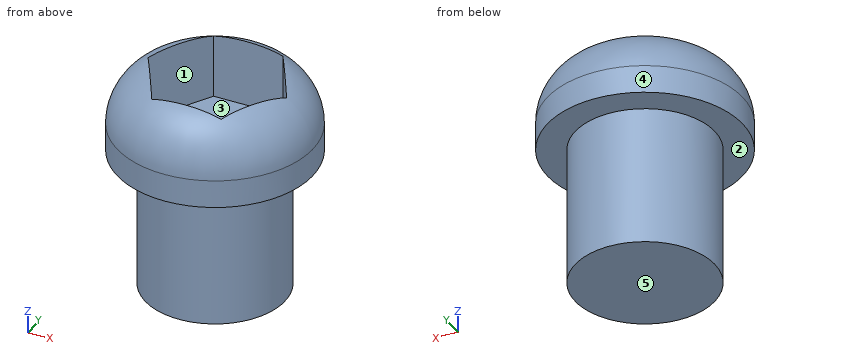
```python
from build123d import *

# Parameters (mm, degrees)
SKETCH1_R           = 3.5
BOSS_EXTRUDE1_DEPTH = 3
SKETCH2_R           = 2.5
BOSS_EXTRUDE2_DEPTH = 5
CUT_EXTRUDE2_DEPTH  = 2.5
FILLET3_R           = 2


with BuildPart() as part:
    # Sketch1 → Boss-Extrude1 (new body)
    with BuildSketch(Plane.XY):
        with Locations((-3.184162196, -0.348949282)):
            Circle(SKETCH1_R)
    extrude(amount=BOSS_EXTRUDE1_DEPTH)

    # Sketch2 → Boss-Extrude2 (add)
    with BuildSketch(Plane(origin=(0, 0, 0), x_dir=(-1, 0, 0), z_dir=(0, 0, -1))):
        with Locations((3.184162196, -0.348949282)):
            Circle(SKETCH2_R)
    extrude(amount=BOSS_EXTRUDE2_DEPTH)

    # Sketch3 → Cut-Extrude2 (cut)
    with BuildSketch(Plane.XY.offset(3)):
        Polygon((-4.340417486, 1.812146916), (-5.592559216, -0.341272384), (-4.353714262, -2.502368582), (-1.862727578, -2.510045479), (-0.610585848, -0.356626179), (-1.849430802, 1.804470018), align=None)
    extrude(amount=-CUT_EXTRUDE2_DEPTH, mode=Mode.SUBTRACT)

    # Fillet3
    # the kernel refuses this fillet: 2 mm, written as the material it takes off along each edge
    with BuildSketch(Plane(origin=(-3.184162196, -0.348949282, 3), x_dir=(1, 0, 0), z_dir=(0, -1, 0))) as fillet3_piece_1:
        with BuildLine():
            CenterArc((3.5 - FILLET3_R, -FILLET3_R), FILLET3_R, 0, 90)
            Line((3.5 - FILLET3_R, 0), (3.5, 0))
            Line((3.5, 0), (3.5, -FILLET3_R))
        make_face()
    revolve(axis=Axis((-3.184162196, -0.348949282, 3), (0, 0, 1)), mode=Mode.SUBTRACT)


solid = part.part
```
Geometry: final body of the model. Coordinates: model frame, mm. Face numbers are marked on the shaded views. A direction names the side the tool comes from. Round coordinates to 2 decimals unless told otherwise and drop trailing zeros. Loops run counter-clockwise (first coordinate to the right, second up) from the corner with the lowest first, then second, coordinate; pieces in that order, holes last. Notation, with made-up numbers: (40, 43) -> (54, 43) arc R24 ccw to (54, 54) -> close; hole circle Ø4 at (33, -16). An arc over 180 degrees is marked (long way). Use one line per item in the form item = value. Start each with the question number.
1) Access query for the marked faces 1 and 2. Directions: +Z, -Z, +X, -X, +Y, -Y. A direction counts if a zero-diameter tool reaches every point of the face in a straight line with its end or side. Return the directions, or none.
2) First-contact query: P1, Ø4, axis at x = -0.5, y = -1.5, coming from the -Z side; P2, Ø2, axis at x = -3, y = 0.5, coming from the +Z side; P3, Ø3, axis at x = -2.5, y = 1, coming from the +Z side. Flat tips, straight axial feed; report the tip coordinate or a pass-through.
3) Section A-A on z = -3.25. Output: boundary loops of the cut face in (x, y).
4) Line query: L1, parallel to Z at x = -1.5, y = -1.25; L2, parallel to Y at x = -3.25, z = -4.5; L3, parallel to X at y = 1.5, z = 2. Output: solid intervals per line, ascending.
5) Draft query along Y for the marked faces 3, 4 and 5. Return one class per face: released by +Y, released by -Y, zero draft, split by the parting line, or undercut.
Response:
q1.face_1 = +Z
q1.face_2 = -Z
q2.P1 = -5
q2.P2 = 0.5
q2.P3 = 2.89
q3.outline = circle Ø5 at (-3.18, -0.35)
q4.L1 = -5 to 0.5
q4.L2 = -2.85 to 2.15
q4.L3 = -5.84 to -4.52, -1.67 to -0.53
q5.face_3 = undercut
q5.face_4 = split by the parting line
q5.face_5 = zero draft
